```python
from build123d import *

# Parameters (mm, degrees)
EXTRUDE_1_DEPTH     = 9
SKETCH_2_R          = 3.5
CUT_EXTRUDE_1_DEPTH = 18
EXTRUDE_2_DEPTH     = 10
EXTRUDE_START       = 2.5
SKETCH_4_R          = 3.5
EXTRUDE_3_DEPTH     = 2.5
CHAMFER_1_SIZE      = 1
EXTRUDE_5_DEPTH     = 10
SKETCH_7_W          = 65.185315269
SKETCH_7_H          = 30.661532817
CUT_EXTRUDE_2_DEPTH = 10


with BuildPart() as part:
    # 草图1 → 凸台-拉伸1 (new, symmetric)
    with BuildSketch(Plane.XY):
        with BuildLine():
            Line((-38.810889132, -2.777568136), (-8.5, 14.722431864))
            ThreePointArc((-8.5, 14.722431864), (-1.481647627, 16.935309868), (5.814342437, 15.974774553))
            Line((5.814342437, 15.974774553), (6.498382723, 17.854159795))
            ThreePointArc((6.498382723, 17.854159795), (-1.655959112, 18.927699264), (-9.5, 16.454482672))
            Line((-9.5, 16.454482672), (-39.810889132, -1.045517328))
            Line((-39.810889132, -1.045517328), (-38.810889132, -2.777568136))
        make_face()
    extrude(amount=EXTRUDE_1_DEPTH, both=True)

    # 草图2 → 切除-拉伸1 (cut)
    with BuildSketch(Plane(origin=(-9.5, 16.454482672, 0), x_dir=(0.8660254037844398, 0.49999999999999806, 0), z_dir=(-0.49999999999999806, 0.8660254037844398, 0))):
        with Locations(Location((-26, 0, 0), (0, 0, 180))):
            Circle(SKETCH_2_R)
    extrude(amount=-CUT_EXTRUDE_1_DEPTH, mode=Mode.SUBTRACT)

    # 草图7 → 切除-拉伸2 (cut, symmetric)
    with BuildSketch(Plane.XY):
        with Locations((-14.546201846, 8.806087934)):
            Rectangle(SKETCH_7_W, SKETCH_7_H)
    extrude(amount=CUT_EXTRUDE_2_DEPTH, both=True, mode=Mode.SUBTRACT)


with BuildPart() as body_2:
    # 草图3 → 凸台-拉伸2 (new, symmetric)
    with BuildSketch(Plane.XY):
        Polygon((-26, 4.618802154), (-26, -73), (-41, -73), (-41, -4.041451884), align=None)
    extrude(amount=EXTRUDE_2_DEPTH, both=True)

    # 草图4 → 凸台-拉伸3 (add)
    with BuildSketch(Plane(origin=(-8.5, 14.722431864, 0), x_dir=(0.8660254037844386, 0.5000000000000001, 0), z_dir=(-0.5000000000000001, 0.8660254037844386, 0)).offset(EXTRUDE_START)):
        with Locations((-26, 0)):
            Circle(SKETCH_4_R)
    extrude(amount=-EXTRUDE_3_DEPTH)

    # 倒角1
    chamfer_1_edges = [body_2.edges().sort_by_distance(p)[0] for p in [
        (-35.297749412, 2.137495374, 0),
    ]]
    chamfer(chamfer_1_edges, length=CHAMFER_1_SIZE)

    # 草图6 → 凸台-拉伸5 (add, symmetric)
    with BuildSketch(Plane.XY):
        Polygon((-38.810889132, -2.777568136), (-39.310889132, -1.911542732), (-41, -2.886751346), (-41, -4.041451884), align=None)
    extrude(amount=EXTRUDE_5_DEPTH, both=True)


solid = body_2.part
```
Verification items for the finished model (mm, model axes). Round coordinates to 2 decimals unless told otherwise and drop trailing zeros. Write each loop counter-clockwise with the first axis right and the second up, starting at its lowest first coordinate (ties: lowest second). Pieces come first, ordered by that corner, then holes. Notation, with made-up numbers: (36, -11.5) - (93, -11.5) arc R12 ccw to (93, 1.5) - close; hole circle Ø8 at (22, 46.25). An arc over 180 degrees is marked (long way). Answer as a JSON object with one key per item and string values. Group by question number.
Q1. Thickness scan on line 1 (Y direction, x = -28, z = -1); line 2 (Y direction, x = -31, z = -5); line 3 (X direction, y = 0, z = 0). Record the ranges inside material, lowest first.
Q2. Section check A-A, the plane z = -8. Enter the section's corners in (x, y).
Q3. Go/stop test with a flat-tipped pin: pin 1 Ø3 at (x, z) = (-30.5, -5) entering from +Y. Record where the tip stops, or that it passes through.
Q4. Mould release check, pull along X, two halves, no side actions. Record for faces 1 (the flat face through (-34, -34, 10)), 2 (the flat face through (-40.14, -2.39, 0.14)), 3 (the flat face through (-34, 0, -2)), 4 (the cylindrical face through (-28.6, 4, 1.34)): released by +X, released by -X, zero draft, split by the parting line, or undercut.
Q5. Section check B-B, the plane x = -37. Enter the section's corners in (y, z), plus the area to 3 significant figures.
Found:
{
 "1": {"line 1": "y = -73 to 3.46", "line 2": "y = -73 to 1.73", "line 3": "x = -34.06 to -26"},
 "2": {"outline": "(-41, -73) - (-26, -73) - (-26, 4.62) - (-38.81, -2.78) - (-39.31, -1.91) - (-41, -2.89) - close"},
 "3": {"pin 1": "stops at y = 2.89"},
 "4": {"face 1": "zero draft", "face 2": "released by -X", "face 3": "undercut", "face 4": "undercut"},
 "5": {"outline": "(-73, -10) - (-1.73, -10) - (-1.73, 10) - (-73, 10) - close", "area": "1,430 mm^2"}
}
